Answer from the drawing. Dimensions are ordinates in mm from the lowest x, y and z of the part. A direction names the side the tool comes from. Coordinates: 2 decimals unless noted, no trailing zeros. Order: outer loops, then holes, each group sorted by start corner. A loop starts at its lowest first (then second) coordinate and runs counter-clockwise, first axis right, second up. Notation, with made-up numbers: (32, 53.5) - (73, 53.5) arc R21 cw to (73, 67.5) - close; hole circle Ø8 at (62, 84). An arc over 180 degrees is marked (long way). Answer as a JSON object with one key per item and string values. Group by question number.
1) The mould has two halves that part along Z. Classify the marked faces 6, 7 and 8: released by +Z, released by -Z, zero draft, split by the parting line, or undercut.
2) Find the intervals of material crossed by line 1 along X through (y, z) = (4.75, 3.25); line 2 along X through (y, z) = (2.75, 5.5); line 3 along Y through (x, z) = (23, 6.25), in increasing order.
3) Section C-C (z = 4.25) is taken. Give the vertices of the cut face in (x, y).
4) Section A-A (y = 1.5) is taken. Count the separate pieces of the cut face and the enclosed holes in it.
5) Section B-B (x = 7.75) is taken. Give the vertices of the cut face in (y, z), plus the area to 3 significant figures.
6) Each of these flat-tipped pins is pushed along its axis until it touches: P1, Ø1.6, axis at x = 4, z = 4.5, coming from the +Y side; P2, Ø2, axis at y = 10, z = 4, coming from the -X side; P3, Ø1, axis at y = 5.5, z = 2, coming from the +X side. Where does it stop, or does it pass through?
7) A tool of negligible diameter and unlimited length cuts with its end or side. For the marked faces 1, 2, 3, 4 and 5, from which of +Z, -Z, +X, -X, +Y, -Y can it reach the whole face along a straight path? Write none if from no direction.
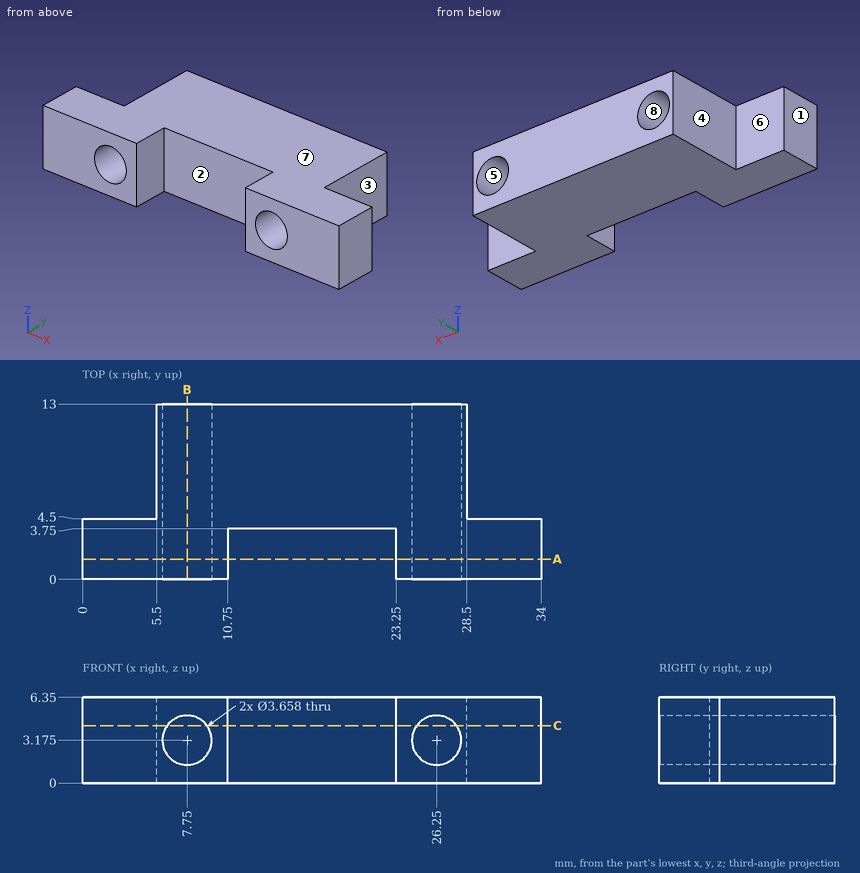
Report:
{
 "1": {"face 6": "zero draft", "face 7": "released by +Z", "face 8": "undercut"},
 "2": {"line 1": "x = 5.5 to 5.92, 9.58 to 24.42, 28.08 to 28.5", "line 2": "x = 0 to 10.75, 23.25 to 34", "line 3": "y = 3.75 to 13"},
 "3": {"outline": "(0, 0) - (6.27, 0) - (6.27, 13) - (5.5, 13) - (5.5, 4.5) - (0, 4.5) - close; (9.23, 0) - (10.75, 0) - (10.75, 3.75) - (23.25, 3.75) - (23.25, 0) - (24.77, 0) - (24.77, 13) - (9.23, 13) - close; (27.73, 0) - (34, 0) - (34, 4.5) - (28.5, 4.5) - (28.5, 13) - (27.73, 13) - close"},
 "4": {"separate pieces": "2", "enclosed holes": "2"},
 "5": {"outline": "(0, 0) - (13, 0) - (13, 1.35) - (0, 1.35) - close; (0, 5) - (13, 5) - (13, 6.35) - (0, 6.35) - close", "area": "35.0 mm²"},
 "6": {"P1": "stops at y = 4.5", "P2": "stops at x = 5.5", "P3": "stops at x = 28.5"},
 "7": {"face 1": "+Z, -Z, -X, +Y, -Y", "face 2": "+Z, -Z, -Y", "face 3": "+Z, -Z, +X, +Y", "face 4": "+Z, -Z, -X, +Y", "face 5": "+Y, -Y"}
}
